Autodesk Inventor part; units mm, degrees
ref_plane "YZ Plane" through (0, 0, 0) normal (1, 0, 0) x (0, 1, 0)
ref_plane "XZ Plane" through (0, 0, 0) normal (0, 1, 0) x (-1, 0, 0)
ref_plane "XY Plane" through (0, 0, 0) normal (0, 0, 1) x (1, 0, 0)
sketch "Skizze1" plane through (0, 0, 0) normal (1, 0, 0) x (0, 1, 0)
  line L0 (0, 0) -> (144, 0)
  line L1 (144, 0) -> (144, -68)
  line L2 (144, -68) -> (0, -68)
  line L3 (0, -68) -> (0, 0)
  dimension "d0" = 144
  dimension "d1" = 68
extrude "Extrusion1" add sketch "Skizze1" along normal blind 16
sketch "Skizze2" plane through (0, 0, 0) normal (0, 0, 1) x (1, 0, 0)
  line L0 (0, 0) -> (0, 144) construction
  line L1 (0, 72) -> (16, 72) construction
  line L2 (16, 144) -> (16, 0) construction
  line L3 (0, 144) -> (16, 144) construction
  line L4 (8, 144) -> (8, 0) construction
  line L5 (0, 144) -> (16, 144) construction
  line L6 (0, 0) -> (16, 0) construction
  line L7 (0, 144) -> (16, 144) construction
  line L8 (16, 144) -> (16, 0) construction
  line L9 (16, 0) -> (0, 0) construction
  line L10 (0, 0) -> (0, 144) construction
  line L11 (0, 112) -> (16, 112) construction
  line L12 (0, 32) -> (16, 32) construction
  point P0 (8, 112)
  point P1 (8, 72)
  point P2 (8, 32)
  dimension "d4" = 40
  dimension "d5" = 40
hole "Bohrung1" at (8, 112, 0) at (8, 72, 0) at (8, 32, 0) direction (0, 0, -1) diameter 3 depth 30 tip angle 118
sketch "Skizze3" plane through (0, 144, 0) normal (0, 1, 0) x (1, 0, 0)
  line L0 (0, 0) -> (16, 0)
  line L1 (16, 0) -> (16, 68)
  line L2 (16, 68) -> (0, 68)
  line L3 (0, 68) -> (0, 0)
  line L4 (8, 0) -> (8, 68) construction
  line L5 (0, 68) -> (16, 68) construction
  line L6 (16, 0) -> (16, 68) construction
  line L7 (16, 34) -> (0, 34) construction
  line L8 (0, 68) -> (0, 0) construction
  line L9 (0, 14) -> (16, 14) construction
  line L10 (0, 54) -> (16, 54) construction
  point P0 (8, 14)
  point P1 (8, 54)
  dimension "d13" = 14
  dimension "d22" = 14
hole "Bohrung2" at (8, 144, -14) at (8, 144, -54) direction (0, -1, 0) diameter 3 depth 25 tip angle 118
sketch "Skizze4" plane through (0, 0, -68) normal (0, 0, -1) x (-1, 0, 0)
  line L0 (0, 0) -> (-16, 0) construction
  line L1 (-16, 0) -> (-16, 144) construction
  line L2 (-16, 144) -> (0, 144) construction
  line L3 (0, 144) -> (0, 0) construction
  line L4 (-8, 0) -> (-8, 144) construction
  line L5 (-16, 144) -> (-16, 0) construction
  line L6 (-16, 72) -> (0, 72) construction
  circle A0 centre (-8, 72) radius 1.5 construction
  point P0 (-8, 112)
  point P1 (-8, 32)
  dimension "d23" = 40
  dimension "d24" = 40
hole "Bohrung3" at (8, 72, -68) at (8, 112, -68) at (8, 32, -68) direction (0, 0, 1) diameter 3 depth 30 tip angle 118
sketch "Skizze5" plane through (16, 0, 0) normal (1, 0, 0) x (0, 0, -1)
  line L0 (68, 144) -> (0, 144) construction
  line L1 (0, 144) -> (0, 0) construction
  line L2 (0, 0) -> (68, 0) construction
  line L3 (68, 0) -> (68, 144) construction
  line L4 (0, 144) -> (0, 0) construction
  line L5 (0, 72) -> (68, 72) construction
  circle A0 centre (34, 72) radius 4 construction
  line L6 (20, 119) -> (20, 39) construction
  point P0 (20, 79)
  dimension "d41" = 8
  dimension "d42" = 7
  dimension "d43" = 40
  dimension "d44" = 40
  dimension "d45" = 20
hole "Bohrung4" at (16, 39, -20) at (16, 79, -20) at (16, 119, -20) direction (-1, 0, 0) diameter 3 end through all countersink diameter 8 countersink angle 90
hole "Bohrung5" at (16, 72, -34) direction (-1, 0, 0) diameter 8 end through all
equation "\"d39\" = Stärke"
equation "\"d51\" = Stärke"
equation "\"Biegeradius\" = Stärke"
equation "\"BreiteBiegungsfreistellung\" = Stärke"
equation "\"TiefeBiegungsfreistellung\" = 0.5 * Stärke"
equation "\"GrößeEckenfreistellung\" = 4 * Stärke"
equation "\"MinimalRest\" = 2 * Stärke"
equation "\"Übergangsradius\" = Biegeradius"
equation "\"JacobiRadiusGröße\" = Biegeradius"
equation "\"Abstandsgröße\" = Stärke"
properties part number "licht_200_side_right"
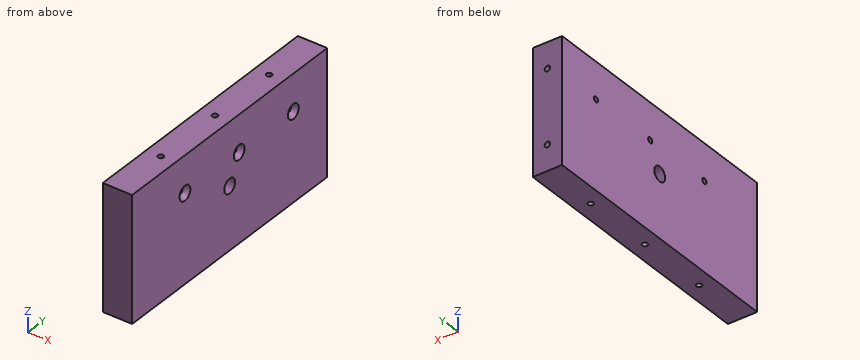
Source: CAD feature listing. Evaluate the final solid. Frame: model axes, mm. Round coordinates to 2 decimals unless told otherwise and drop trailing zeros. Loops run counter-clockwise (first coordinate to the right, second up) from the corner with the lowest first, then second, coordinate; pieces in that order, holes last. Notation, with made-up numbers: (44.5, 80.25) - (67.5, 80.25) arc R23 cw to (67.5, 113.25) - close; hole circle Ø1 at (11.25, 19). An arc over 180 degrees is marked (long way). Write item = value, one per line. Start each with the question number.
Item 1: Material intervals for line 1 (Y direction, x = 8, z = -22.75); line 2 (X direction, y = 112, z = -49); line 3 (Y direction, x = 8.5, z = -49), sorted ascending.
Item 2: First-contact query: pin 1 Ø2.5 at (x, y) = (8, 32) entering from +Z; pin 2 Ø2.5 at (x, y) = (8, 72) entering from -Z; pin 3 Ø4 at (y, z) = (119, -20) entering from +X. Flat tips, straight axial feed; report the tip coordinate or a pass-through.
Item 3: Section query A-A on z = -20. Output: boundary loops of the cut face in (x, y), plus the area to 3 significant figures.
Item 4: Section query B-B on y = 39. Output: boundary loops of the cut face in (x, z).
Results list:
q1.line_1 = 0 to 30.5, 33.5 to 70.5, 73.5 to 110.5, 113.5 to 144
q1.line_2 = 0 to 6.5, 9.5 to 16
q1.line_3 = 0 to 30.59, 33.41 to 70.59, 73.41 to 110.59, 113.41 to 144
q2.pin_1 = -30.15
q2.pin_2 = -37.85
q2.pin_3 = 14
q3.outline = (0, 0) - (16, 0) - (16, 35) - (13.5, 37.5) - (0, 37.5) - close; (0, 40.5) - (13.5, 40.5) - (16, 43) - (16, 75) - (13.5, 77.5) - (0, 77.5) - close; (0, 80.5) - (13.5, 80.5) - (16, 83) - (16, 115) - (13.5, 117.5) - (0, 117.5) - close; (0, 120.5) - (13.5, 120.5) - (16, 123) - (16, 144) - (0, 144) - close; hole circle Ø3 at (8, 32); hole circle Ø3 at (8, 72); hole circle Ø3 at (8, 112)
q3.area = 2,120 mm²
q4.outline = (0, -68) - (16, -68) - (16, -24) - (13.5, -21.5) - (0, -21.5) - close; (0, -18.5) - (13.5, -18.5) - (16, -16) - (16, 0) - (0, 0) - close
